from build123d import *

# Parameters (mm, degrees)
SKETCH1_R           = 10.5
BOSS_EXTRUDE1_DEPTH = 6
SKETCH2_R           = 1.25
CUT_EXTRUDE1_DEPTH  = 17.015617378
SKETCH3_W           = 3.5
SKETCH3_H           = 7.7
CUT_EXTRUDE2_DEPTH  = 6


with BuildPart() as part:
    # Sketch1 → Boss-Extrude1 (new body)
    with BuildSketch(Plane(origin=(0, 0, 0), x_dir=(0, 0, -1), z_dir=(1, 0, 0))):
        Circle(SKETCH1_R)
    extrude(amount=BOSS_EXTRUDE1_DEPTH)

    # Sketch2 → Cut-Extrude1 (cut, through all)
    with BuildSketch(Plane(origin=(6, 0, 0), x_dir=(0, 0, -1), z_dir=(1, 0, 0))):
        with Locations((0, 8)):
            Circle(SKETCH2_R)
        with Locations((6.92820323, 4)):
            Circle(SKETCH2_R)
        with Locations((6.92820323, -4)):
            Circle(SKETCH2_R)
        with Locations((0, -8)):
            Circle(SKETCH2_R)
        with Locations((-6.92820323, -4)):
            Circle(SKETCH2_R)
        with Locations((-6.92820323, 4)):
            Circle(SKETCH2_R)
    extrude(amount=-CUT_EXTRUDE1_DEPTH, mode=Mode.SUBTRACT)

    # Sketch3 → Cut-Extrude2 (cut)
    with BuildSketch(Plane(origin=(6, 0, 0), x_dir=(0, 0, -1), z_dir=(1, 0, 0))):
        Rectangle(SKETCH3_W, SKETCH3_H)
    extrude(amount=-CUT_EXTRUDE2_DEPTH, mode=Mode.SUBTRACT)


solid = part.part
Source: CAD feature listing. Evaluate the final solid. Frame: model axes, mm. A direction names the side the tool comes from. Round coordinates to 2 decimals unless told otherwise and drop trailing zeros. Order: outer loops, then holes, each group sorted by start corner. A loop starts at its lowest first (then second) coordinate and runs counter-clockwise, first axis right, second up. Notation, with made-up numbers: (5.5, -14.75) - (17.5, -14.75) arc R24 ccw to (17.5, 23.25) - close; hole circle Ø7 at (-20.5, -24.5). An arc over 180 degrees is marked (long way). Use a Markdown table: item, result. Add a question column.
1. Set-up query: faces 1 (the flat face through (3, -3.85, 0)), 2 (the flat face through (0, 0, -2)). Return all of +Z, -Z, +X, -X, +Y, -Y with unobstructed straight access to the full face (end or side cutting, diameter ignored); none if empty.
2. Section query C-C (z = 6.25). Return the cut outline in (x, y), then the cut area to 3 significant figures.
3. Section query B-B (y = 0). Return the cut outline in (x, z).
4. Section query D-D (y = 4.25). Return the cut outline in (x, z), then the cut area to 3 significant figures.
5. Mould query, pull axis Z, two halves, no side actions, for faces 3 (the cylindrical face through (3.042, -4.761, -5.936)), 4 (the cylindrical face through (3, 3.2, -10)), 5 (the flat face through (6, 0, -2)). Classes: +Z half, -Z half, draft (parallel to the pull), parting line (faces both ways), or undercut.
6. Line query: probe 1 along Y at (x, z) = (2.6, 0); probe 2 along Y at (x, z) = (3.15, -8); probe 3 along Z at (x, y) = (3.25, 1.25). Output: solid intervals per line, ascending.
7. Section query A-A (x = 2.6). Return the cut outline in (y, z), then the cut area to 3 significant figures.
8. First-contact query: pin 1 (1.5 mm diameter, centred on x = 2, y = -0.5, fed in from +Z); pin 2 (1.8 mm diameter, centred on x = 2.5, y = -1.5, fed in from -Z); pin 3 (2 mm diameter, centred on y = 4, z = -6.93, fed in from +X); pin 4 (2 mm diameter, centred on x = 3.5, y = 7.5, fed in from -Z). Flat tips, straight axial feed; report the tip coordinate or a pass-through.
Derived:
| question | item | result |
|---|---|---|
| 1 | face 1 | +X, -X |
| 1 | face 2 | +Z, -Z, -X, +Y, -Y |
| 2 | outline | (0, -8.44) - (6, -8.44) - (6, -5.05) - (0, -5.05) - close; (0, -2.95) - (6, -2.95) - (6, 2.95) - (0, 2.95) - close; (0, 5.05) - (6, 5.05) - (6, 8.44) - (0, 8.44) - close |
| 2 | area | 76.0 mm2 |
| 3 | outline | (0, -10.5) - (6, -10.5) - (6, -1.75) - (0, -1.75) - close; (0, 1.75) - (6, 1.75) - (6, 10.5) - (0, 10.5) - close |
| 4 | outline | (0, -9.6) - (6, -9.6) - (6, -8.15) - (0, -8.15) - close; (0, -5.7) - (6, -5.7) - (6, 5.7) - (0, 5.7) - close; (0, 8.15) - (6, 8.15) - (6, 9.6) - (0, 9.6) - close |
| 4 | area | 85.8 mm2 |
| 5 | face 3 | undercut |
| 5 | face 4 | parting line |
| 5 | face 5 | draft |
| 6 | probe 1 | -10.5 to -9.25, -6.75 to -3.85, 3.85 to 6.75, 9.25 to 10.5 |
| 6 | probe 2 | -6.8 to -4.64, -3.36 to 3.36, 4.64 to 6.8 |
| 6 | probe 3 | -10.43 to -1.75, 1.75 to 10.43 |
| 7 | outline | circle Ø21 at (0, 0); hole circle Ø2.5 at (-8, 0); hole circle Ø2.5 at (-4, -6.93); hole circle Ø2.5 at (-4, 6.93); hole (-3.85, -1.75) - (3.85, -1.75) - (3.85, 1.75) - (-3.85, 1.75) - close; hole circle Ø2.5 at (4, -6.93); hole circle Ø2.5 at (4, 6.93); hole circle Ø2.5 at (8, 0) |
| 7 | area | 290 mm2 |
| 8 | pin 1 | z = 10.5 |
| 8 | pin 2 | z = -10.48 |
| 8 | pin 3 | through |
| 8 | pin 4 | z = -8.25 |
